from build123d import *


with BuildPart() as part:
    # Esboço1 → Revolução1 (revolve)
    with BuildSketch(Plane.XY, mode=Mode.PRIVATE) as revolu_o1_sk:
        Polygon((0, 4.725), (3.5, 4.725), (3.5, 4.55), (4.85, 4.55), (4.85, 4.725), (8.6, 4.725), (8.6, 5.6), (11.6, 5.6), (11.6, 4.725), (28, 4.725), (28, 4), (0, 4), align=None)
    revolve(revolu_o1_sk.sketch.rotate(Axis((0, 0, 0), (1, 0, 0)), 90), axis=Axis((0, 0, 0), (1, 0, 0)))


solid = part.part
Can you work these out from the model? Positions are in its coordinate system, mm. A direction names the side the tool comes from. Round coordinates to 2 decimals unless told otherwise and drop trailing zeros. Loops run counter-clockwise (first coordinate to the right, second up) from the corner with the lowest first, then second, coordinate; pieces in that order, holes last. Notation, with made-up numbers: (23.25, -34) - (41.25, -34) arc R31 ccw to (41.25, -3) - close; hole circle Ø3 at (12, 18). An arc over 180 degrees is marked (long way). Write item = value, one per line. Start each with the question number.
(1) If I drill on probe 1 along Y at (x, z) = (14, 0) (3 decimals); probe 2 along Y at (x, z) = (8.75, 0); probe 3 along X at (y, z) = (-5, 2), over which ranges is the centre line in solid material (lowest first)? Write a range as [from, to].
(2) For P1, Ø6.5, axis at y = 0, z = 0, coming from the +X side; P2, Ø5, axis at x = 3.5, z = -4.5, coming from the +Y side; P3, Ø6, axis at x = 6, y = 3.5, coming from the -Z side, each with a flat end and sliding along its axis, tell me the tip position at first contact or that it passes through.
(3) For faces 4 (the face through (6.751, -1.419, 4.507)), 5 (the face through (4.18, 2.77, -3.61)), 6 (the face through (28, -2, -4)), 7 (the face through (11.6, 4, -3)), which set-ups out of +Z, -Z, +X, -X, +Y, -Y let a thin tool reach every point of the face, with its end or its side?
(4) If we section it at A-A (z = 0): Please give me the cut outline in (x, y) (3 decimals), and give its area (3 significant figures).
(5) If we section it at C-C (x = 2): Please give me the cut outline in (y, z) (3 decimals), and give its area (3 significant figures).
(6) If we mould it in two halves opening along Z, with no side actions, what happens to faces 1 (the face through (10.121, -0.246, -5.595)), 2 (the face through (13.804, 3.905, -0.867)), 3 (the face through (8.6, 4, 3))? For each: released by +Z, released by -Z, zero draft, split by the parting line, or undercut.
Ans:
q1.probe_1 = [-4.725, -4], [4, 4.725]
q1.probe_2 = [-5.6, -4], [4, 5.6]
q1.probe_3 = [8.6, 11.6]
q2.P1 = through
q2.P2 = 4.28
q2.P3 = -5.23
q3.face_4 = -X
q3.face_5 = none
q3.face_6 = +Z, -Z, +X, +Y, -Y
q3.face_7 = +X
q4.outline = (0, -4.725) - (3.5, -4.725) - (3.5, -4.55) - (4.85, -4.55) - (4.85, -4.725) - (8.6, -4.725) - (8.6, -5.6) - (11.6, -5.6) - (11.6, -4.725) - (28, -4.725) - (28, -4) - (0, -4) - close; (0, 4) - (28, 4) - (28, 4.725) - (11.6, 4.725) - (11.6, 5.6) - (8.6, 5.6) - (8.6, 4.725) - (4.85, 4.725) - (4.85, 4.55) - (3.5, 4.55) - (3.5, 4.725) - (0, 4.725) - close
q4.area = 45.4 mm²
q5.outline = circle Ø9.45 at (0, 0); hole circle Ø8 at (0, 0)
q5.area = 19.9 mm²
q6.face_1 = split by the parting line
q6.face_2 = undercut
q6.face_3 = zero draft
